Design review of the part built by this model. Coordinates are the model's own, in mm. A direction names the side the tool comes from. Give positions to 0.01 mm unless a question says otherwise; leave off trailing zeros. Loops run counter-clockwise (first coordinate to the right, second up) from the corner with the lowest first, then second, coordinate; pieces in that order, holes last. Notation, with made-up numbers: (52.25, 1.5) -> (109.25, 1.5) arc R36 cw to (109.25, 40.5) -> close; hole circle Ø3 at (-34, 87). An arc over 180 degrees is marked (long way). Answer in a Markdown table with one row per item. Add a question column.
(1) For line 1 (Z direction, x = 14.5, y = -4); line 2 (Y direction, x = -3.5, z = 17); line 3 (Z direction, x = -7.5, y = -19), list the stretches that pass through material, from the lowest coordinate up.
(2) Consider section B-B on z = 0. Write out the cut boundary in (x, y), then the cut area to 3 significant figures.
(3) Consider section C-C on x = 0. Write out the cut boundary in (y, z), then the cut area to 3 significant figures.
(4) Consider section D-D on x = -7. Write out the cut boundary in (y, z), then the cut area to 3 significant figures.
(5) Draft analysis for pull direction Y (two halves, no side actions). For faces 4 (the cylindrical face through (-19.077, -16.888, 19.107)), 5 (the flat face through (-21.15, -29, 0)), 6 (the flat face through (-0.1, -25, 20.5)), 7 (the flat face through (0, 24, 0)), state which applies: +Y half, -Y half, draft (parallel to the pull), parting line (faces both ways), or undercut.
(6) For pin 1 (13 mm diameter, centred on x = -5, y = -13.5, fed in from -Z); pin 2 (1.5 mm diameter, centred on x = -15, z = 16, fed in from +Y); pin 3 (1.5 mm diameter, centred on x = -4.5, y = -18, fed in from -Z); pin 4 (12.5 mm diameter, centred on x = 7.5, z = -10, fed in from +Y), all flat-tipped, find the tip position at first contact; note any pin that passes through.
(7) For faces 1 (the cylindrical face through (14.155, -2.218, 16.178)), 2 (the flat face through (2, 13, 0)), 3 (the cylindrical face through (19.8, -4.4, 19.8)), list the 3-axis set-ups (+Z, -Z, +X, -X, +Y, -Y) from which the entire face can be reached by the end or side of a thin tool; tool diameter is ignored.
(8) Consider section A-A on y = -11. Write out the cut boundary in (x, z), then the cut area to 3 significant figures.
from build123d import *

# Parameters (mm, degrees)
BOSS_EXTRUDE1_DEPTH = 24
SKETCH2_R           = 11
BOSS_EXTRUDE2_DEPTH = 2
BOSS_EXTRUDE3_DEPTH = 9
BOSS_EXTRUDE4_DEPTH = 16
BOSS_EXTRUDE5_DEPTH = 9
SKETCH6_R           = 1.5
CUT_EXTRUDE1_DEPTH  = 4.5


with BuildPart() as part:
    # Sketch1 → Boss-Extrude1 (new body)
    with BuildSketch(Plane(origin=(0, 0, 0), x_dir=(1, 0, 0), z_dir=(0, 1, 0))):
        with BuildLine():
            Line((2, 1.5), (2, -1.5))
            ThreePointArc((2, -1.5), (-2.5, 0), (2, 1.5))
        make_face()
    extrude(amount=BOSS_EXTRUDE1_DEPTH)

    # Sketch2 → Boss-Extrude2 (add)
    with BuildSketch(Plane(origin=(0, 0, 0), x_dir=(1, 0, 0), z_dir=(0, 1, 0))):
        with Locations(Location((0, 0, 0), (0, 0, 270))):
            Circle(SKETCH2_R)
    extrude(amount=BOSS_EXTRUDE2_DEPTH)

    # Sketch3 → Boss-Extrude3 (add)
    with BuildSketch(Plane(origin=(0, 0, 0), x_dir=(1, 0, 0), z_dir=(0, 1, 0))):
        with BuildLine():
            Line((-18.348773801, 21.15), (18.348773801, 21.15))
            ThreePointArc((18.348773801, 21.15), (19.798989873, 19.798989873), (21.15, 18.348773801))
            Line((21.15, 18.348773801), (21.15, -18.348773801))
            ThreePointArc((21.15, -18.348773801), (19.798989873, -19.798989873), (18.348773801, -21.15))
            Line((18.348773801, -21.15), (-18.348773801, -21.15))
            ThreePointArc((-18.348773801, -21.15), (-19.798989873, -19.798989873), (-21.15, -18.348773801))
            Line((-21.15, -18.348773801), (-21.15, 18.348773801))
            ThreePointArc((-21.15, 18.348773801), (-19.798989873, 19.798989873), (-18.348773801, 21.15))
        make_face()
    extrude(amount=-BOSS_EXTRUDE3_DEPTH)

    # Sketch4 → Boss-Extrude4 (add)
    with BuildSketch(Plane.XZ.offset(9)):
        with BuildLine():
            Line((20.15, -17.971574778), (20.15, 17.971574778))
            ThreePointArc((20.15, 17.971574778), (19.091883092, 19.091883092), (17.971574778, 20.15))
            Line((17.971574778, 20.15), (-17.971574778, 20.15))
            ThreePointArc((-17.971574778, 20.15), (-19.091883092, 19.091883092), (-20.15, 17.971574778))
            Line((-20.15, 17.971574778), (-20.15, -17.971574778))
            ThreePointArc((-20.15, -17.971574778), (-19.091883092, -19.091883092), (-17.971574778, -20.15))
            Line((-17.971574778, -20.15), (17.971574778, -20.15))
            ThreePointArc((17.971574778, -20.15), (19.091883092, -19.091883092), (20.15, -17.971574778))
        make_face()
    extrude(amount=BOSS_EXTRUDE4_DEPTH)

    # Sketch5 → Boss-Extrude5 (add)
    with BuildSketch(Plane.XZ.offset(25)):
        with BuildLine():
            Line((21.15, -18.348773801), (21.15, 18.348773801))
            ThreePointArc((21.15, 18.348773801), (19.798989873, 19.798989873), (18.348773801, 21.15))
            Line((18.348773801, 21.15), (-18.348773801, 21.15))
            ThreePointArc((-18.348773801, 21.15), (-19.798989873, 19.798989873), (-21.15, 18.348773801))
            Line((-21.15, 18.348773801), (-21.15, -18.348773801))
            ThreePointArc((-21.15, -18.348773801), (-19.798989873, -19.798989873), (-18.348773801, -21.15))
            Line((-18.348773801, -21.15), (18.348773801, -21.15))
            ThreePointArc((18.348773801, -21.15), (19.798989873, -19.798989873), (21.15, -18.348773801))
        make_face()
    extrude(amount=BOSS_EXTRUDE5_DEPTH)

    # Sketch6 → Cut-Extrude1 (cut)
    with BuildSketch(Plane(origin=(0, 0, 0), x_dir=(1, 0, 0), z_dir=(0, 1, 0))):
        with Locations(Location((-15.485638508, 15.485638508, 0), (0, 0, 270))):
            Circle(SKETCH6_R)
        with Locations(Location((15.485638508, 15.485638508, 0), (0, 0, 270))):
            Circle(SKETCH6_R)
        with Locations(Location((15.485638508, -15.485638508, 0), (0, 0, 270))):
            Circle(SKETCH6_R)
        with Locations(Location((-15.485638508, -15.485638508, 0), (0, 0, 270))):
            Circle(SKETCH6_R)
    extrude(amount=-CUT_EXTRUDE1_DEPTH, mode=Mode.SUBTRACT)


solid = part.part
Values follow:
| question | item | result |
|---|---|---|
| 1 | line 1 | -21.15 to -16.62, -14.35 to 14.35, 16.62 to 21.15 |
| 1 | line 2 | -34 to 0 |
| 1 | line 3 | -20.15 to 20.15 |
| 2 | outline | (-21.15, -34) -> (21.15, -34) -> (21.15, -25) -> (20.15, -25) -> (20.15, -9) -> (21.15, -9) -> (21.15, 0) -> (11, 0) -> (11, 2) -> (2, 2) -> (2, 24) -> (-2.5, 24) -> (-2.5, 2) -> (-11, 2) -> (-11, 0) -> (-21.15, 0) -> (-21.15, -9) -> (-20.15, -9) -> (-20.15, -25) -> (-21.15, -25) -> close |
| 2 | area | 1,550 mm2 |
| 3 | outline | (-34, -21.15) -> (-25, -21.15) -> (-25, -20.15) -> (-9, -20.15) -> (-9, -21.15) -> (0, -21.15) -> (0, -11) -> (2, -11) -> (2, -2.5) -> (24, -2.5) -> (24, 2.5) -> (2, 2.5) -> (2, 11) -> (0, 11) -> (0, 21.15) -> (-9, 21.15) -> (-9, 20.15) -> (-25, 20.15) -> (-25, 21.15) -> (-34, 21.15) -> close |
| 3 | area | 1,560 mm2 |
| 4 | outline | (-34, -21.15) -> (-25, -21.15) -> (-25, -20.15) -> (-9, -20.15) -> (-9, -21.15) -> (0, -21.15) -> (0, -8.49) -> (2, -8.49) -> (2, 8.49) -> (0, 8.49) -> (0, 21.15) -> (-9, 21.15) -> (-9, 20.15) -> (-25, 20.15) -> (-25, 21.15) -> (-34, 21.15) -> close |
| 4 | area | 1,440 mm2 |
| 5 | face 4 | undercut |
| 5 | face 5 | draft |
| 5 | face 6 | undercut |
| 5 | face 7 | +Y half |
| 6 | pin 1 | z = -21.15 |
| 6 | pin 2 | y = -4.5 |
| 6 | pin 3 | z = -20.15 |
| 6 | pin 4 | y = 2 |
| 7 | face 1 | +Y |
| 7 | face 2 | +Z, -Z, +X, +Y |
| 7 | face 3 | +Z, +X, +Y, -Y |
| 8 | outline | (-20.15, -17.97) arc R27 ccw to (-17.97, -20.15) -> (17.97, -20.15) arc R27 ccw to (20.15, -17.97) -> (20.15, 17.97) arc R27 ccw to (17.97, 20.15) -> (-17.97, 20.15) arc R27 ccw to (-20.15, 17.97) -> close |
| 8 | area | 1,610 mm2 |
